CAD build for the part. Positions are in the model's coordinates, mm. Face numbers are marked on the shaded views. Coordinates: 2 decimals unless noted, no trailing zeros. Order: outer loops, then holes, each group sorted by start corner. A loop starts at its lowest first (then second) coordinate and runs counter-clockwise, first axis right, second up. Notation, with made-up numbers: (-24, -34.5) - (-10, -34.5) arc R17 ccw to (-10, -19.5) - close; hole circle Ø8 at (54, 50). An arc over 180 degrees is marked (long way). Return JSON: item names as keys, results as strings.
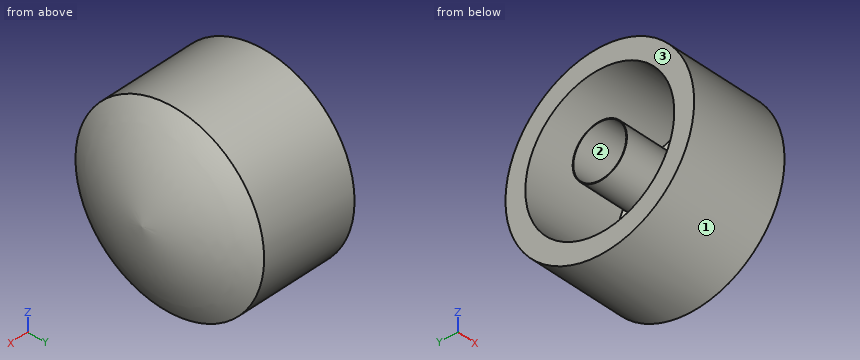
from build123d import *

# Parameters (mm, degrees)
F0_W     = 15
F0_H     = 3
F2_R     = 4.1
F4_R     = 4
F5_DEPTH = 11


with BuildPart() as f1:
    # F0 (on Top) → F1 (revolve)
    with BuildSketch(Plane.XY):
        with Locations((7.5, 12.75)):
            Rectangle(F0_W, F0_H)
        with BuildLine():
            ThreePointArc((19.6392323583, 0), (18.1392323583, 7.3918343789), (15, 14.25))
            Line((15, 14.25), (15, 11.25))
            ThreePointArc((15, 11.25), (16.9445632196, 5.7296263006), (18.1392323583, 0))
            Line((18.1392323583, 0), (19.6392323583, 0))
        make_face()
    revolve(axis=Axis((16.0183925182, 0, 0), (1, 0, 0)))

    # F2 (on Right) → F3 (join, up to the next surface of F1)
    with BuildSketch(Plane.YZ):
        Circle(F2_R)
    extrude(until=Until.NEXT)

    # F4 (on face) → F5 (cut)
    with BuildSketch(Plane(origin=(0, 0, 0), x_dir=(0, -1, 0), z_dir=(-1, 0, 0))):
        Circle(F4_R)
    extrude(amount=-F5_DEPTH, mode=Mode.SUBTRACT)


solid = f1.part
Item 1: Band-saw the part on C-C, the plane x = 16.75. Count the separate pieces of the cut face and the enclosed holes in it, then the cut area to 3 significant figures.
Findings below:
{"separate pieces": "2", "enclosed holes": "1", "area": "300 mm²"}
Item 2: Wall check: L1, parallel to Z at x = 11.5, y = -1.5; L2, parallel to Z at x = 14, y = 2.5; L3, parallel to Z at x = 10, y = -6. Give the ranges that are in metal, low to high. Write a range as [from, to].
Findings below:
{"L1": "z = [-14.17, -11.15], [-3.82, 3.82], [11.15, 14.17]", "L2": "z = [-14.03, -10.97], [-3.25, 3.25], [10.97, 14.03]", "L3": "z = [-12.93, -9.52], [9.52, 12.93]"}
Item 3: Band-saw the part on A-A, the plane x = 14.5. List the corners of the cut face in (y, z).
Findings below:
{"outline": "circle Ø28.5 at (0, 0); circle Ø8.2 at (0, 0); hole circle Ø22.5 at (0, 0)"}
Item 4: Band-saw the part on B-B, the plane x = 2.75. List the corners of the cut face in (y, z).
Findings below:
{"outline": "circle Ø28.5 at (0, 0); circle Ø8.2 at (0, 0); hole circle Ø22.5 at (0, 0); hole circle Ø8 at (0, 0)"}
Item 5: Drop flat-ended pins along their axis: P1, Ø4, axis at x = 2.5, y = 6, coming from the -Z side; P2, Ø10, axis at x = 10, z = 6, coming from the -Y side; P3, Ø1, axis at y = 7.5, z = 7, coming from the +X side. Give the stop position or say it passes through.
Findings below:
{"P1": "stops at z = -13.68", "P2": "stops at y = -14.21", "P3": "stops at x = 17.27"}
Item 6: Mould opens along Z. For the marked faces 1, 2 and 3 say: released by +Z, released by -Z, zero draft, split by the parting line, or undercut.
Findings below:
{"face 1": "split by the parting line", "face 2": "undercut", "face 3": "zero draft"}
